Here's how the part is built. I have some questions about the finished solid (model axes, mm). A direction names the side the tool comes from. Give positions to 0.01 mm unless a question says otherwise; leave off trailing zeros. Loops run counter-clockwise (first coordinate to the right, second up) from the corner with the lowest first, then second, coordinate; pieces in that order, holes last.
Q1. If we section it at B-B (y = 3): Please give me the cut outline in (x, z) (3 decimals).
Q2. If we section it at A-A (y = -2.25): Please give me the cut outline in (x, z) (3 decimals).
Q3. If we section it at D-D (z = 2): Please give me the cut outline in (x, y) (3 decimals), plus the area to 3 significant figures.
Q4. We'd pull the mould along X, two halves only. Please class faces 5 (the face through (24.375, -4, 5)), 6 (the face through (0, 6.5, 5)), 7 (the face through (-18.5, -6.5, 4.9)): +X half, -X half, draft (parallel to the pull), parting line (faces both ways), or undercut.
Q5. Will these pins go through, and if not, where does the flat tip stop? P1, Ø3.5, axis at x = -20.2, z = 5, coming from the +Y side; P2, Ø2.5, axis at x = 20.2, z = 5, coming from the +Y side; P3, Ø5, axis at x = -3, z = 6.5, coming from the -Y side; P4, Ø5, axis at y = 4, z = 3.5, coming from the -X side (3 decimals).
Q6. For faces 1 (the face through (22, -1.5, 5)), 2 (the face through (-23.924, -3.965, 0.428)), 3 (the face through (-22, -1.5, 5)), 4 (the face through (-11.803, -6.049, 5.07)), which set-ups out of +Z, -Z, +X, -X, +Y, -Y let a thin tool reach every point of the face, with its end or its side?
Q7. If we section it at C-C (z = 5): Please give me the cut outline in (x, y) (3 decimals).
Q8. I need wall thicknesses on line 1 (X direction, y = 2.5, z = 9.5) (3 decimals); line 2 (X direction, y = -2.25, z = 4.25) (1 decimal); line 3 (Y direction, x = 9.5, z = 3.25). Which ranges of each line are inside material? Lowest first, please.
from build123d import *

# Parameters (mm, degrees)
BOSS_EXTRU_1_DEPTH      = 10
ESQUISSE2_W             = 10
ESQUISSE2_H             = 5
BOSS_EXTRU_2_DEPTH      = 8
ESQUISSE3_W             = 10
ESQUISSE3_H             = 5
BOSS_EXTRU_3_DEPTH      = 8
CONG_1_R                = 1.5
CONG_2_R                = 1.5
ESQUISSE4_R             = 1.5
ENL_V_MAT_EXTRU_1_DEPTH = 30.379255011


with BuildPart() as part:
    # Esquisse1 → Boss.-Extru.1 (new body)
    with BuildSketch(Plane.XY):
        with BuildLine():
            ThreePointArc((-16.375, 9), (-15.642766953, 10.767766953), (-13.875, 11.5))
            Line((-13.875, 11.5), (13.875, 11.5))
            ThreePointArc((13.875, 11.5), (15.642766953, 10.767766953), (16.375, 9))
            Line((16.375, 9), (16.375, -6.5))
            Line((16.375, -6.5), (11.375, -6.5))
            Line((11.375, -6.5), (11.375, 6.5))
            Line((11.375, 6.5), (-11.375, 6.5))
            Line((-11.375, 6.5), (-11.375, -6.5))
            Line((-11.375, -6.5), (-16.375, -6.5))
            Line((-16.375, -6.5), (-16.375, 9))
        make_face()
    extrude(amount=BOSS_EXTRU_1_DEPTH)

    # Esquisse2 → Boss.-Extru.2 (add)
    with BuildSketch(Plane.ZY.offset(16.375)):
        with Locations((5, -4)):
            Rectangle(ESQUISSE2_W, ESQUISSE2_H)
    extrude(amount=BOSS_EXTRU_2_DEPTH)

    # Esquisse3 → Boss.-Extru.3 (add)
    with BuildSketch(Plane(origin=(16.375, 0, 0), x_dir=(0, 0, -1), z_dir=(1, 0, 0))):
        with Locations((-5, -4)):
            Rectangle(ESQUISSE3_W, ESQUISSE3_H)
    extrude(amount=BOSS_EXTRU_3_DEPTH)

    # Congé1
    cong_1_edges = [part.edges().sort_by_distance(p)[0] for p in [
        (-24.375, -4, 0),
        (-24.375, -4, 10),
        (24.375, -4, 10),
        (24.375, -4, 0),
    ]]
    fillet(cong_1_edges, radius=CONG_1_R)

    # Congé2
    cong_2_edges = [part.edges().sort_by_distance(p)[0] for p in [
        (11.375, -6.5, 5),
        (-11.375, -6.5, 5),
    ]]
    fillet(cong_2_edges, radius=CONG_2_R)

    # Esquisse4 → Enlèv. mat.-Extru.1 (cut, through all)
    with BuildSketch(Plane(origin=(0, -1.5, 0), x_dir=(1, 0, 0), z_dir=(0, 1, 0))):
        with Locations(Location((-20.198529412, -5, 0), (0, 0, 180))):
            Circle(ESQUISSE4_R)
        with Locations(Location((20.198529412, -5, 0), (0, 0, 180))):
            Circle(ESQUISSE4_R)
    extrude(amount=-ENL_V_MAT_EXTRU_1_DEPTH, mode=Mode.SUBTRACT)


solid = part.part
Check sheet entries:
1. outline: (-16.375, 0) - (-11.375, 0) - (-11.375, 10) - (-16.375, 10) - close; (11.375, 0) - (16.375, 0) - (16.375, 10) - (11.375, 10) - close
2. outline: (-24.375, 1.5) arc R1.5 ccw to (-22.875, 0) - (-11.375, 0) - (-11.375, 10) - (-22.875, 10) arc R1.5 ccw to (-24.375, 8.5) - close; (11.375, 0) - (22.875, 0) arc R1.5 ccw to (24.375, 1.5) - (24.375, 8.5) arc R1.5 ccw to (22.875, 10) - (11.375, 10) - close; hole circle Ø3 at (-20.199, 5); hole circle Ø3 at (20.199, 5)
3. outline: (-24.375, -6.5) - (-12.875, -6.5) arc R1.5 ccw to (-11.375, -5) - (-11.375, 6.5) - (11.375, 6.5) - (11.375, -5) arc R1.5 ccw to (12.875, -6.5) - (24.375, -6.5) - (24.375, -1.5) - (16.375, -1.5) - (16.375, 9) arc R2.5 ccw to (13.875, 11.5) - (-13.875, 11.5) arc R2.5 ccw to (-16.375, 9) - (-16.375, -1.5) - (-24.375, -1.5) - close
3. area: 370 mm2
4. face 5: +X half
4. face 6: undercut
4. face 7: draft
5. P1: stops at y = -1.5
5. P2: passes through
5. P3: stops at y = 6.5
5. P4: stops at x = -16.375
6. face 1: +Z, -Z, +X, +Y
6. face 2: -Z, -X, +Y, -Y
6. face 3: +Z, -Z, -X, +Y
6. face 4: +Z, -Z, -Y
7. outline: (-24.375, -6.5) - (-21.699, -6.5) - (-21.699, -1.5) - (-24.375, -1.5) - close; (-18.699, -6.5) - (-12.875, -6.5) arc R1.5 ccw to (-11.375, -5) - (-11.375, 6.5) - (11.375, 6.5) - (11.375, -5) arc R1.5 ccw to (12.875, -6.5) - (18.699, -6.5) - (18.699, -1.5) - (16.375, -1.5) - (16.375, 9) arc R2.5 ccw to (13.875, 11.5) - (-13.875, 11.5) arc R2.5 ccw to (-16.375, 9) - (-16.375, -1.5) - (-18.699, -1.5) - close; (21.699, -6.5) - (24.375, -6.5) - (24.375, -1.5) - (21.699, -1.5) - close
8. line 1: x = -16.375 to -11.375, 11.375 to 16.375
8. line 2: x = -24.4 to -21.5, -18.9 to -11.4, 11.4 to 18.9, 21.5 to 24.4
8. line 3: y = 6.5 to 11.5
